Design review of the part built by this model. Coordinates are the model's own, in mm. Face numbers are marked on the shaded views. Give positions to 0.01 mm unless a question says otherwise; leave off trailing zeros. Write each loop counter-clockwise with the first axis right and the second up, starting at its lowest first coordinate (ties: lowest second). Pieces come first, ordered by that corner, then holes. Notation, with made-up numbers: (85, -37) -> (109, -37) arc R24 cw to (109, -12) -> close; hole circle Ø4 at (-7.5, -1). An arc over 180 degrees is marked (long way). Return JSON: item names as keys, results as strings. Group by question number.
from build123d import *

# Parameters (mm, degrees)
F0_R     = 82.9945
F0_R_2   = 7.9375
F0_R_3   = 20.6375
F0_R_4   = 4.7625
F1_DEPTH = 25
F2_D     = 6.7564
F3_DEPTH = 6.35
F5_D     = 10.71626


# Not quite as in the source:
# - a feature names something its author has since deleted; it is built from what else it names


with BuildPart() as f1:
    # F0 (on Front) → F1 (new body)
    with BuildSketch(Plane.XZ):
        Circle(F0_R)
        with Locations((-23.0087746099, -50.5745756008)):
            Circle(F0_R_2, mode=Mode.SUBTRACT)
        with Locations((-40.9891773098, -37.5110483686)):
            Circle(F0_R_2, mode=Mode.SUBTRACT)
        with Locations((23.0087746099, -50.5745756008)):
            Circle(F0_R_2, mode=Mode.SUBTRACT)
        with Locations((40.9891773098, -37.5110483686)):
            Circle(F0_R_2, mode=Mode.SUBTRACT)
        with Locations((-55.2093820582, 6.2542416807)):
            Circle(F0_R_2, mode=Mode.SUBTRACT)
        with Locations((-48.3414793582, 27.3914727554)):
            Circle(F0_R_2, mode=Mode.SUBTRACT)
        with Locations((-11.1125, 54.4399095334)):
            Circle(F0_R_2, mode=Mode.SUBTRACT)
        Circle(F0_R_3, mode=Mode.SUBTRACT)
        with Locations((55.2093820582, 6.2542416807)):
            Circle(F0_R_2, mode=Mode.SUBTRACT)
        with Locations((48.3414793582, 27.3914727554)):
            Circle(F0_R_2, mode=Mode.SUBTRACT)
        with Locations((11.1125, 54.4399095334)):
            Circle(F0_R_2, mode=Mode.SUBTRACT)
        with Locations((-48.3414793582, 27.3914727554)):
            Circle(F0_R_2)
        with Locations((-48.3414793582, 27.3914727554)):
            Circle(F0_R_4, mode=Mode.SUBTRACT)
        with Locations((-11.1125, 54.4399095334)):
            Circle(F0_R_2)
        with Locations((-11.1125, 54.4399095334)):
            Circle(F0_R_4, mode=Mode.SUBTRACT)
        with Locations((-55.2093820582, 6.2542416807)):
            Circle(F0_R_2)
        with Locations((-55.2093820582, 6.2542416807)):
            Circle(F0_R_4, mode=Mode.SUBTRACT)
        with Locations((-40.9891773098, -37.5110483686)):
            Circle(F0_R_2)
        with Locations((-40.9891773098, -37.5110483686)):
            Circle(F0_R_4, mode=Mode.SUBTRACT)
        with Locations((-23.0087746099, -50.5745756008)):
            Circle(F0_R_2)
        with Locations((-23.0087746099, -50.5745756008)):
            Circle(F0_R_4, mode=Mode.SUBTRACT)
        with Locations((55.2093820582, 6.2542416807)):
            Circle(F0_R_2)
        with Locations((55.2093820582, 6.2542416807)):
            Circle(F0_R_4, mode=Mode.SUBTRACT)
        with Locations((48.3414793582, 27.3914727554)):
            Circle(F0_R_2)
        with Locations((48.3414793582, 27.3914727554)):
            Circle(F0_R_4, mode=Mode.SUBTRACT)
        with Locations((11.1125, 54.4399095334)):
            Circle(F0_R_2)
        with Locations((11.1125, 54.4399095334)):
            Circle(F0_R_4, mode=Mode.SUBTRACT)
        with Locations((23.0087746099, -50.5745756008)):
            Circle(F0_R_2)
        with Locations((23.0087746099, -50.5745756008)):
            Circle(F0_R_4, mode=Mode.SUBTRACT)
        with Locations((40.9891773098, -37.5110483686)):
            Circle(F0_R_2)
        with Locations((40.9891773098, -37.5110483686)):
            Circle(F0_R_4, mode=Mode.SUBTRACT)
        with Locations((-55.2093820582, 6.2542416807)):
            Circle(F0_R_4)
        with Locations((-40.9891773098, -37.5110483686)):
            Circle(F0_R_4)
        with Locations((-23.0087746099, -50.5745756008)):
            Circle(F0_R_4)
        with Locations((55.2093820582, 6.2542416807)):
            Circle(F0_R_4)
        with Locations((48.3414793582, 27.3914727554)):
            Circle(F0_R_4)
        with Locations((11.1125, 54.4399095334)):
            Circle(F0_R_4)
    extrude(amount=F1_DEPTH)

    # F2 (through all)
    with Locations(Plane(origin=(0, 0, 0), x_dir=(1, 0, 0), z_dir=(0, 1, 0))):
        with Locations((0, -69.85), (41.0567998726, -56.5098370571), (66.4312976632, -21.5848370571), (66.4312976632, 21.5848370571), (41.0567998726, 56.5098370571), (0, 69.85), (-41.0567998726, 56.5098370571), (-66.4312976632, 21.5848370571), (-66.4312976632, -21.5848370571), (-41.0567998726, -56.5098370571)):
            Hole(F2_D / 2)

    # F0 (on Front) → F3 (cut)
    with BuildSketch(Plane.XZ):
        with Locations((-11.1125, 54.4399095334)):
            Circle(F0_R_2)
        with Locations((-11.1125, 54.4399095334)):
            Circle(F0_R_4, mode=Mode.SUBTRACT)
        with Locations((-48.3414793582, 27.3914727554)):
            Circle(F0_R_2)
        with Locations((-48.3414793582, 27.3914727554)):
            Circle(F0_R_4, mode=Mode.SUBTRACT)
        with Locations((40.9891773098, -37.5110483686)):
            Circle(F0_R_2)
        with Locations((40.9891773098, -37.5110483686)):
            Circle(F0_R_4, mode=Mode.SUBTRACT)
        with Locations((23.0087746099, -50.5745756008)):
            Circle(F0_R_2)
        with Locations((23.0087746099, -50.5745756008)):
            Circle(F0_R_4, mode=Mode.SUBTRACT)
    extrude(amount=F3_DEPTH, mode=Mode.SUBTRACT)

    # F5 (through all)
    with Locations(Plane(origin=(0, 0, 0), x_dir=(1, 0, 0), z_dir=(0, 1, 0))):
        with Locations((0, 45), (42.7975432333, 13.9057647469), (26.4503363532, -36.4057647469), (-26.4503363532, -36.4057647469), (-42.7975432333, 13.9057647469)):
            Hole(F5_D / 2)


solid = f1.part
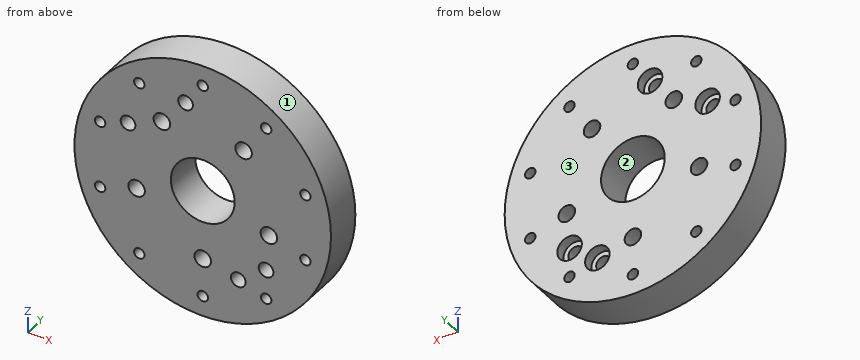
Q1. Take a section at B-B, the plane z = 0. Give the boundary of the cut face in (x, y), plus the area to 3 significant figures.
Q2. Take a section at C-C, the plane y = -16.5. Count the separate pieces of the cut face and the enclosed holes in it, plus the area to 3 significant figures.
Q3. Take a section at A-A, the plane x = 0. Give the boundary of the cut face in (y, z).
Q4. Mouldability with a two-part tool opening along X and no side actions: class the marked faces 1, 2 and 3 as +X half, -X half, draft (parallel to the pull), parting line (faces both ways), or undercut.
Q5. For L1, parallel to Z at x = 0, y = -6.25; L2, parallel to X at y = -10.25, z = 31.5; L3, parallel to Z at x = 46, y = -5.75, list the stretches that pass through material, from the lowest coordinate up. Write a range as from..to.
Q6. Take a section at D-D, the plane z = 69.85. Give the boundary of the cut face in (x, y).
Q7. Insertion check: pin 1 (5 mm diameter, centred on y = -20, z = -17.5, fed in from -X); pin 2 (11 mm diameter, centred on x = 41.06, z = 56.51, fed in from -Y); pin 3 (3 mm diameter, centred on y = -4.5, z = 60.5, fed in from -X); pin 4 (1 mm diameter, centred on y = -10, z = 60.5, fed in from -X). Each pin has a flat end and moves straight along its axis. Give the tip position at first contact, or say it passes through.
Final values:
{
 "1": {"outline": "(-82.99, -25) -> (-20.64, -25) -> (-20.64, 0) -> (-82.99, 0) -> close; (20.64, -25) -> (82.99, -25) -> (82.99, 0) -> (20.64, 0) -> close", "area": "3,120 mm²"},
 "2": {"separate pieces": "1", "enclosed holes": "20", "area": "19,200 mm²"},
 "3": {"outline": "(-25, -82.99) -> (0, -82.99) -> (0, -73.23) -> (-25, -73.23) -> close; (-25, -66.47) -> (0, -66.47) -> (0, -50.36) -> (-25, -50.36) -> close; (-25, -39.64) -> (0, -39.64) -> (0, -20.64) -> (-25, -20.64) -> close; (-25, 20.64) -> (0, 20.64) -> (0, 66.47) -> (-25, 66.47) -> close; (-25, 73.23) -> (0, 73.23) -> (0, 82.99) -> (-25, 82.99) -> close"},
 "4": {"face 1": "parting line", "face 2": "undercut", "face 3": "draft"},
 "5": {"L1": "z = -82.99..-73.23, -66.47..-50.36, -39.64..-20.64, 20.64..66.47, 73.23..82.99", "L2": "x = -76.78..-50.75, -45.93..-28.61, -24.3..24.3, 28.61..76.78", "L3": "z = -69.08..-43.67, -31.36..-18.2, -9.61..69.08"},
 "6": {"outline": "(-44.82, -25) -> (-3.38, -25) -> (-3.38, 0) -> (-44.82, 0) -> close; (3.38, -25) -> (44.82, -25) -> (44.82, 0) -> (3.38, 0) -> close"},
 "7": {"pin 1": "stops at x = -81.63", "pin 2": "stops at y = -25", "pin 3": "stops at x = -58.37", "pin 4": "stops at x = -57.34"}
}
